Autodesk Inventor part; units mm, degrees
ref_plane "YZ Plane" through (0, 0, 0) normal (1, 0, 0) x (0, 1, 0)
ref_plane "XZ Plane" through (0, 0, 0) normal (0, 1, 0) x (-1, 0, 0)
ref_plane "XY Plane" through (0, 0, 0) normal (0, 0, 1) x (1, 0, 0)
sketch "Esboço1" plane through (0, 0, 0) normal (1, 0, 0) x (0, 1, 0)
  line L0 (10.9206, 18.8054) -> (-21.8794, 18.8054)
  line L1 (-21.8794, 18.8054) -> (-21.8794, 2.1054)
  line L2 (-21.8794, 2.1054) -> (10.9206, 2.1054)
  line L3 (10.9206, 2.1054) -> (10.9206, 18.8054)
  circle A0 centre (4.3506, 9.8054) radius 3.25
  circle A1 centre (4.3506, 9.8054) radius 3.8294
  circle A2 centre (-5.1194, 9.8054) radius 3.25
  circle A3 centre (-5.1194, 9.8054) radius 3.8763
  circle A4 centre (-14.5894, 9.8054) radius 3.25
  circle A5 centre (-14.5894, 9.8054) radius 3.9245
  point P0 (0, 0)
  point P1 (-5.4794, 18.8054)
  dimension "d0" = 32.8
  dimension "d1" = 16.7
  dimension "d2" = 32.8
  dimension "d7" = 6.5
  dimension "d8" = 6.5
  dimension "d9" = 6.5
  dimension "d22" = 9
  dimension "d23" = 9
  dimension "d24" = 9
extrude "Extrusão1" add sketch "Esboço1" along normal blind 3 contours L3 L2 L1 L0
sketch "Esboço2" plane through (0, -21.8794, 18.8054) normal (0, 0, 1) x (1, 0, 0)
  line L0 (3, 0) -> (3, 32.8)
  line L1 (0, 32.8) -> (3, 32.8)
  line L2 (3, 32.8) -> (15, 32.8)
  line L3 (15, 32.8) -> (15, 0)
  line L4 (15, 0) -> (3, 0)
  point P0 (0, 21.8794)
  dimension "d13" = 12
extrude "Extrusão2" add sketch "Esboço2" against normal blind 2
sketch "Esboço3" plane through (0, -21.8794, 16.8054) normal (0, 0, -1) x (-1, 0, 0)
  line L0 (0, 32.8) -> (-3, 32.8)
  line L1 (0, 32.8) -> (-15, 32.8)
  line L2 (-3, 32.8) -> (-15, 32.8)
  line L3 (-15, 32.8) -> (-15, 0.0164)
  line L4 (-15, 0.0164) -> (-3, 0.0164)
  point P0 (0, 21.8794)
sketch "Esboço4" plane through (0, -21.8794, 2.1054) normal (0, 0, -1) x (-1, 0, 0)
  line L0 (0, 32.8) -> (-3, 32.8)
  line L1 (0, 32.8) -> (-15, 32.8)
  line L2 (-15, 32.8) -> (-15, 0)
  line L3 (-15, 32.8) -> (-15, 0)
  line L4 (-15, 0) -> (0, 0)
  line L5 (0, 32.8) -> (0, 0)
  line L6 (0, 0) -> (0, 32.8)
  point P0 (0, 21.8794)
extrude "Extrusão3" add sketch "Esboço4" along normal blind 2
sketch "Esboço5" plane through (0, 10.9206, 18.8054) normal (0, 1, 0) x (1, 0, 0)
  line L0 (0, 0) -> (15, 0)
  line L1 (15, 18.7) -> (0, 18.7)
  line L2 (15, 0) -> (15, 18.7)
  line L3 (15, 18.7) -> (0, 18.8054)
  line L4 (0, 18.8054) -> (0, 0)
  line L5 (0, 0) -> (15, 0)
  point P0 (0, 18.7)
extrude "Extrusão4" add sketch "Esboço5" along normal blind 2 contours L4 L1 L2 L0
sketch "Esboço6" plane through (15, -21.8794, 18.8054) normal (1, 0, 0) x (0, 0, -1)
  line L0 (0, 34.8) -> (18.7, 34.8)
  line L1 (0, 0) -> (0, 34.8)
  line L2 (0, 34.8) -> (0, 0)
  line L3 (0, 0) -> (18.7, 0)
  line L4 (18.7, 0) -> (18.7, 34.8)
  line L5 (18.7, 0) -> (18.7, 34.8)
  line L6 (18.7, 34.8) -> (0, 34.8)
  point P0 (18.8054, 21.8794)
extrude "Extrusão5" add sketch "Esboço6" along normal blind 2
sketch "Esboço7" plane through (0, -21.8794, 18.8054) normal (0, 0, 1) x (1, 0, 0)
  point P0 (0, 21.8794)
properties part number "semaforoEsboço"
Could you check a few things on this model? Use its own coordinates, in mm. A direction names the side the tool comes from. Coordinates: 2 decimals unless noted, no trailing zeros. Order: outer loops, then holes, each group sorted by start corner. A loop starts at its lowest first (then second) coordinate and runs counter-clockwise, first axis right, second up. Notation, with made-up numbers: (46.5, 64) - (87.5, 64) arc R33 cw to (87.5, 98) - close; hole circle Ø6 at (-9.75, 75). An arc over 180 degrees is marked (long way). Answer in a Markdown table with one row per item. Add a question column.
(1) If we mould it in two halves opening along X, with no side actions, what happens to faces 4 (the face through (0, -1, 9)), 5 (the face through (2.7, -21.879, 9.6)), 6 (the face through (9, -5, 16.805))? For each: released by +X, released by -X, zero draft, split by the parting line, or undercut.
(2) I need wall thicknesses on L1, parallel to X at y = 1.5, z = 13.5; L2, parallel to Z at x = 10.25, y = -13; L3, parallel to Y at x = 1.75, z = 6.5. Which ranges of each line are inside material? Lowest first, please.
(3) If we section it at B-B, the plane z = 12.5: Please give me the cut outline in (x, y).
(4) Will these pins go through, and if not, where does the flat tip stop? pin 1 (5 mm diameter, centred on x = 5, z = 3.5, fed in from -Y); pin 2 (6 mm diameter, centred on x = 8.5, z = 13, fed in from -Y).
(5) If we section it at C-C, the plane x = 7.5: Please give me the cut outline in (y, z).
(6) If we section it at D-D, the plane z = 16: Please give me the cut outline in (x, y).
(7) On a 3-axis mill with a long thin cutter (end or side, diameter ignored), from which of +Z, -Z, +X, -X, +Y, -Y can I reach the whole of each face in a straight line? I mean faces 1 (the face through (8, -5, 18.805)), 2 (the face through (3, -9.4, 9.6)), 3 (the face through (1.48, 3.85, 6.01)). Say none if no direction works.
(8) If we section it at A-A, the plane y = -19: Please give me the cut outline in (x, z).
Results are:
| question | item | result |
|---|---|---|
| 1 | face 4 | released by -X |
| 1 | face 5 | zero draft |
| 1 | face 6 | undercut |
| 2 | L1 | x = 0 to 3, 15 to 17 |
| 2 | L2 | z = 0.11 to 2.11, 16.81 to 18.81 |
| 2 | L3 | y = -21.88 to -16.71, -12.47 to -7.14, -3.09 to 2.42, 6.28 to 12.92 |
| 3 | outline | (0, -21.88) - (3, -21.88) - (3, -17.44) - (0, -17.44) - close; (0, -11.74) - (3, -11.74) - (3, -7.91) - (0, -7.91) - close; (0, -2.33) - (3, -2.33) - (3, 1.63) - (0, 1.63) - close; (0, 7.07) - (3, 7.07) - (3, 10.92) - (15, 10.92) - (15, -21.88) - (17, -21.88) - (17, 12.92) - (0, 12.92) - close |
| 4 | pin 1 | stops at y = -21.88 |
| 4 | pin 2 | stops at y = 10.92 |
| 5 | outline | (-21.88, 0.11) - (12.92, 0.11) - (12.92, 18.81) - (-21.88, 18.81) - (-21.88, 16.81) - (10.92, 16.81) - (10.92, 2.11) - (-21.88, 2.11) - close |
| 6 | outline | (0, -21.88) - (3, -21.88) - (3, 10.92) - (15, 10.92) - (15, -21.88) - (17, -21.88) - (17, 12.92) - (0, 12.92) - close |
| 7 | face 1 | +Z, +X, -X, +Y, -Y |
| 7 | face 2 | -Y |
| 7 | face 3 | -X |
| 8 | outline | (0, 0.11) - (17, 0.11) - (17, 18.81) - (0, 18.81) - close; hole (3, 2.11) - (15, 2.11) - (15, 16.81) - (3, 16.81) - close |
